from build123d import *

# Parameters (mm, degrees)
F1_DEPTH = 20
F2_R     = 24
F3_DEPTH = 40
F4_R     = 12
F5_DEPTH = 40.001


with BuildPart() as f1:
    # F0 (on Top) → F1 (new body)
    with BuildSketch(Plane.XY):
        with BuildLine():
            Line((112, 24), (0, 24))
            ThreePointArc((0, 24), (-24, 0), (0, -24))
            Line((0, -24), (112, -24))
            ThreePointArc((112, -24), (136, 0), (112, 24))
        make_face()
    extrude(amount=F1_DEPTH)

    # F2 (on Top) → F3 (join)
    with BuildSketch(Plane.XY):
        Circle(F2_R)
    extrude(amount=F3_DEPTH)

    # F4 (on Top) → F5 (cut, through all)
    with BuildSketch(Plane.XY):
        Circle(F4_R)
        with BuildLine():
            Line((109.649421, 12), (57.649421, 12))
            ThreePointArc((57.649421, 12), (45.649421, 0), (57.649421, -12))
            Line((57.649421, -12), (109.649421, -12))
            ThreePointArc((109.649421, -12), (121.649421, 0), (109.649421, 12))
        make_face()
    extrude(amount=F5_DEPTH, mode=Mode.SUBTRACT)


solid = f1.part
Input: part model. Units: mm. Frame: model coordinates. A direction names the side the tool comes from. Coordinates: 2 decimals unless noted, no trailing zeros. Loops run counter-clockwise (first coordinate to the right, second up) from the corner with the lowest first, then second, coordinate; pieces in that order, holes last. Notation, with made-up numbers: (-33, 71.5) - (2, 71.5) arc R27 cw to (2, 101.5) - close; hole circle Ø1 at (0, -8). An arc over 180 degrees is marked (long way). Answer in a Markdown table with one row per item. Add a question column.
Item 1: Line query: line 1 along X through (y, z) = (0, 8); line 2 along X through (y, z) = (0, 22). Output: solid intervals per line, ascending. Write a range as [from, to].
Item 2: Contact query for flat-ended pins moving along their axis: P1, Ø3, axis at y = 4.5, z = 10.5, coming from the -X side; P2, Ø14.5, axis at x = 69, y = -8, coming from the +Z side; P3, Ø10, axis at y = -6, z = 15, coming from the +X side. Output: stop coordinate, or through.
Item 3: Mould query, pull axis X, two halves, no side actions, for faces 4 (the flat face through (84, 12, 10)), 5 (the cylindrical face through (135.994, -0.528, 9.86)), 6 (the flat face through (57, 24, 10)). Classes: released by +X, released by -X, zero draft, split by the parting line, or undercut.
Item 4: Section query C-C on y = 0. Return the cut outline in (x, z), then the cut area to 3 significant figures.
Item 5: Section query A-A on x = 96. Return the cut outline in (y, z).
Item 6: Access query for faces 1 (the cylindrical face through (-23.977, 1.055, 24.164)), 2 (the flat face through (83, -12, 10)), 3 (the flat face through (55, -24, 10)). Directions: +Z, -Z, +X, -X, +Y, -Y. A direction counts if a zero-diameter tool reaches every point of the face in a straight line with its end or side. Return the directions, or none.
Item 7: Section query B-B on z = 16. Return the cut outline in (x, y), then the cut area to 3 significant figures.
Item 8: Section query D-D on z = 28.5. Return the cut outline in (x, y).
Recorded:
| question | item | result |
|---|---|---|
| 1 | line 1 | [-24, -12], [12, 45.65], [121.65, 136] |
| 1 | line 2 | [-24, -12], [12, 24] |
| 2 | P1 | x = -23.81 |
| 2 | P2 | z = 20 |
| 2 | P3 | x = 135.98 |
| 3 | face 4 | undercut |
| 3 | face 5 | released by +X |
| 3 | face 6 | zero draft |
| 4 | outline | (-24, 0) - (-12, 0) - (-12, 40) - (-24, 40) - close; (12, 0) - (45.65, 0) - (45.65, 20) - (24, 20) - (24, 40) - (12, 40) - close; (121.65, 0) - (136, 0) - (136, 20) - (121.65, 20) - close |
| 4 | area | 1,680 mm^2 |
| 5 | outline | (-24, 0) - (-12, 0) - (-12, 20) - (-24, 20) - close; (12, 0) - (24, 0) - (24, 20) - (12, 20) - close |
| 6 | face 1 | +Z |
| 6 | face 2 | +Z, -Z |
| 6 | face 3 | +Z, -Z, +X, -X, -Y |
| 7 | outline | (0, -24) - (112, -24) arc R24 ccw to (112, 24) - (0, 24) arc R24 ccw to start; hole circle Ø24 at (0, 0); hole (57.65, -12) - (109.65, -12) arc R12 ccw to (109.65, 12) - (57.65, 12) arc R12 ccw to start |
| 7 | area | 5,030 mm^2 |
| 8 | outline | circle Ø48 at (0, 0); hole circle Ø24 at (0, 0) |
